from build123d import *

# Parameters (mm, degrees)
SKETCH1_R           = 25.4
BOSS_EXTRUDE1_DEPTH = 76.2
BOSS_EXTRUDE2_DEPTH = 12.7
SKETCH3_R           = 3.175
BOSS_EXTRUDE3_DEPTH = 12.7


with BuildPart() as part:
    # Sketch1 → Boss-Extrude1 (new body)
    with BuildSketch(Plane.XY):
        with Locations(Location((0, 0, 0), (0, 0, 180))):
            Circle(SKETCH1_R)
    extrude(amount=BOSS_EXTRUDE1_DEPTH)

    # Sketch2 → Boss-Extrude2 (add)
    with BuildSketch(Plane.XY.offset(76.2)):
        with BuildLine():
            ThreePointArc((25.4, 0), (0, 25.4), (-25.4, 0))
            Line((-25.4, 0), (25.4, 0))
        make_face()
        with BuildLine():
            Line((25.4, 0), (-25.4, 0))
            ThreePointArc((-25.4, 0), (0, -25.4), (25.4, 0))
        make_face()
        with BuildLine():
            Line((-25.4, 38.1), (-25.4, 0))
            ThreePointArc((-25.4, 0), (0, 25.4), (25.4, 0))
            Line((25.4, 0), (25.4, 38.1))
            Line((25.4, 38.1), (-25.4, 38.1))
        make_face()
    extrude(amount=BOSS_EXTRUDE2_DEPTH)

    # Sketch3 → Boss-Extrude3 (add)
    with BuildSketch(Plane(origin=(0, 0, 0), x_dir=(-1, 0, 0), z_dir=(0, 0, -1))):
        with Locations(Location((0, 0, 0), (0, 0, 180))):
            Circle(SKETCH3_R)
    extrude(amount=BOSS_EXTRUDE3_DEPTH)


solid = part.part
Geometry: final body of the model. Coordinates: model frame, mm. A direction names the side the tool comes from. Coordinates: 2 decimals unless noted, no trailing zeros. Order: outer loops, then holes, each group sorted by start corner. A loop starts at its lowest first (then second) coordinate and runs counter-clockwise, first axis right, second up.
(1) Section query C-C (z = 55). Return the cut outline in (x, y), plus the area to 3 significant figures.
(2) First-contact query: pin 1 (10 mm diameter, centred on x = 3, z = 15, fed in from +Y); pin 2 (11.5 mm diameter, centred on x = -2, y = 12, fed in from -Z); pin 3 (6 mm diameter, centred on x = -7.5, z = 41.5, fed in from -Y). Flat tips, straight axial feed; report the tip coordinate or a pass-through.
(3) Access query for faces 1 (the face through (3.307, -25.184, 43.828)), 2 (the face through (0, 28, 76.2)), 3 (the face through (0, 0, -12.7)). Directions: +Z, -Z, +X, -X, +Y, -Y. A direction counts if a zero-diameter tool reaches every point of the face in a straight line with its end or side. Return the directions, or none.
(4) Section query D-D (y = 17.5). Return the cut outline in (x, z).
(5) Section query B-B (y = 9). Return the cut outline in (x, z).
(6) Section query A-A (x = 0). Return the cut outline in (y, z) (3 decimals), plus the area to 3 significant figures.
(7) Material intervals for probe 1 along Z at (x, y) = (10, 9); probe 2 along Z at (x, y) = (-10, 27.5); probe 3 along Y at (x, z) = (0, 51.5), sorted ascending.
Solution:
1. outline: circle Ø50.8 at (0, 0)
1. area: 2,030 mm2
2. pin 1: stops at y = 25.4
2. pin 2: stops at z = 0
2. pin 3: stops at y = -25
3. face 1: -Z
3. face 2: -Z, +Y
3. face 3: -Z, +X, -X, +Y, -Y
4. outline: (-25.4, 76.2) - (-18.41, 76.2) - (-18.41, 0) - (18.41, 0) - (18.41, 76.2) - (25.4, 76.2) - (25.4, 88.9) - (-25.4, 88.9) - close
5. outline: (-25.4, 76.2) - (-23.75, 76.2) - (-23.75, 0) - (23.75, 0) - (23.75, 76.2) - (25.4, 76.2) - (25.4, 88.9) - (-25.4, 88.9) - close
6. outline: (-25.4, 0) - (-3.175, 0) - (-3.175, -12.7) - (3.175, -12.7) - (3.175, 0) - (25.4, 0) - (25.4, 76.2) - (38.1, 76.2) - (38.1, 88.9) - (-25.4, 88.9) - close
6. area: 4,760 mm2
7. probe 1: z = 0 to 88.9
7. probe 2: z = 76.2 to 88.9
7. probe 3: y = -25.4 to 25.4
